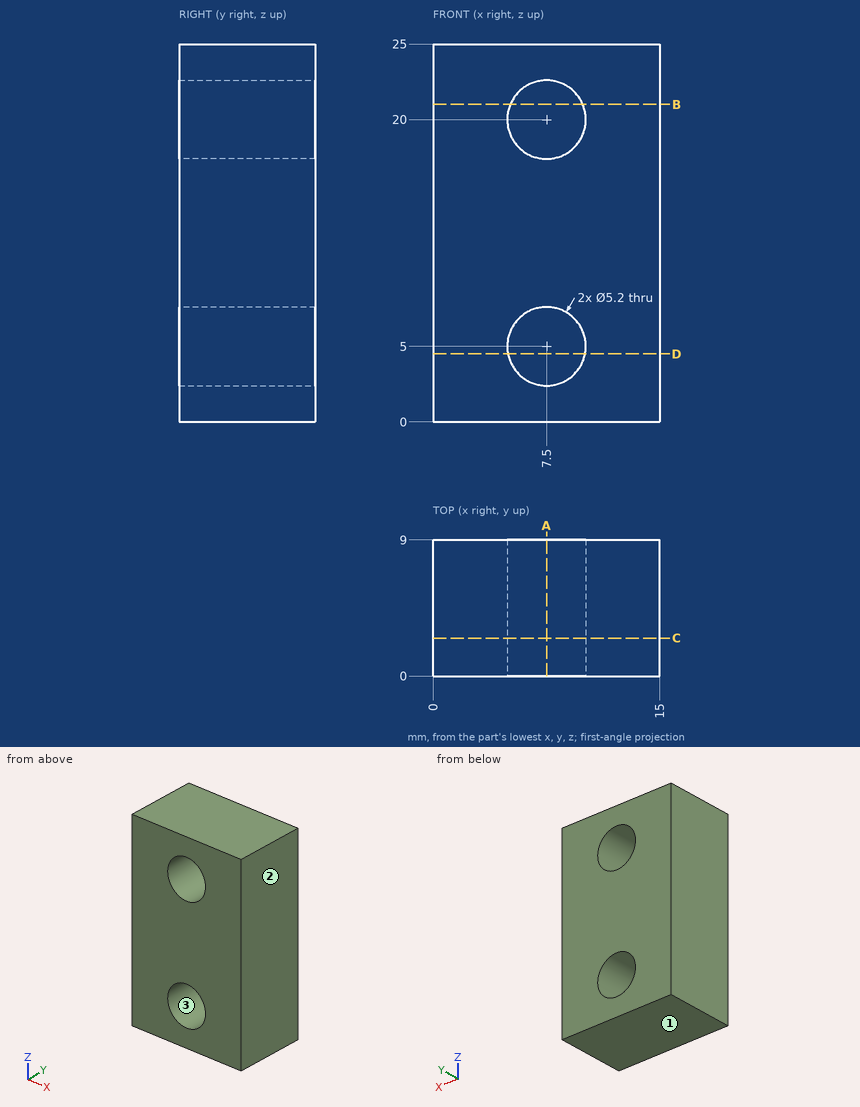
Geometry: see drawing. Coordinates: mm, zero at the bounding-box minimum. Round coordinates to 2 decimals unless told otherwise and drop trailing zeros. Write each loop counter-clockwise with the first axis right and the second up, starting at its lowest first coordinate (ties: lowest second). Pieces come first, ordered by that corner, then holes.
1) Cut plane D-D (z = 4.5). Return the cut outline in (x, y).
2) Cut plane C-C (y = 2.5). Return the cut outline in (x, z).
3) Draft query along X for the marked faces 1, 2 and 3. Return one class per face: pulls with the +X half, pulls with the -X half, needs draft (parallel to the pull), parting line crosses it, or undercut.
4) Cut plane A-A (x = 7.5). Return the cut outline in (y, z).
5) Ray query, L1, parallel to Z at x = 9.5, y = 1; L2, parallel to Z at x = 5.75, y = 4; L3, parallel to X at y = 3.5, z = 20. Return the intervals inside material, ascending.
6) Contact query for a flat-ended pin moving along its axis: P1, Ø4, axis at x = 7.5, z = 5, coming from the -Y side. Output: stop coordinate, or through.
7) Cut plane B-B (z = 21). Return the cut outline in (x, y), then the cut area to 3 significant figures.
Geometry says:
1. outline: (0, 0) - (4.95, 0) - (4.95, 9) - (0, 9) - close; (10.05, 0) - (15, 0) - (15, 9) - (10.05, 9) - close
2. outline: (0, 0) - (15, 0) - (15, 25) - (0, 25) - close; hole circle Ø5.2 at (7.5, 5); hole circle Ø5.2 at (7.5, 20)
3. face 1: needs draft
3. face 2: pulls with the +X half
3. face 3: undercut
4. outline: (0, 0) - (9, 0) - (9, 2.4) - (0, 2.4) - close; (0, 7.6) - (9, 7.6) - (9, 17.4) - (0, 17.4) - close; (0, 22.6) - (9, 22.6) - (9, 25) - (0, 25) - close
5. L1: z = 0 to 3.34, 6.66 to 18.34, 21.66 to 25
5. L2: z = 0 to 3.08, 6.92 to 18.08, 21.92 to 25
5. L3: x = 0 to 4.9, 10.1 to 15
6. P1: passes through
7. outline: (0, 0) - (5.1, 0) - (5.1, 9) - (0, 9) - close; (9.9, 0) - (15, 0) - (15, 9) - (9.9, 9) - close
7. area: 91.8 mm2
